The model under review builds one solid part; all positions refer to its coordinate system, in mm. Face numbers are marked on the shaded views. A direction names the side the tool comes from. Round coordinates to 2 decimals unless told otherwise and drop trailing zeros. Order: outer loops, then holes, each group sorted by start corner. A loop starts at its lowest first (then second) coordinate and runs counter-clockwise, first axis right, second up. Notation, with made-up numbers: M 78,-24.75 L 90,-24.75 A23 cw 90,14.25 Z; hole C 5,-33.75 d1. An arc over 180 degrees is marked long. Use a Markdown table: item, result. Add a question column.
1. The part is to be moulded in two halves that separate along X. For the marked faces 4, 5 and 6, say which applies: +X half, -X half, draft (parallel to the pull), parting line (faces both ways), or undercut.
2. Insertion check: P1, Ø8, axis at y = 15.5, z = 25, coming from the -X side; P2, Ø12.5, axis at x = 15.5, y = 8.5, coming from the +Z side; P3, Ø7.5, axis at y = 8, z = 25, coming from the +X side. Each pin has a flat end and moves straight along its axis. Give the tip position at first contact, or say it passes through.
3. Consider section A-A on x = 57.15. State the section outline as (y, z) points, then the cut area to 3 significant figures.
4. To check wall thickness, follow probe 1 along X at (y, z) = (12.7, 8.75); probe 2 along Y at (x, z) = (57, 9); probe 3 along Z at (x, y) = (3, 20). State the ranges of each line that lie inside material, in increasing order.
5. For the marked faces 1, 2 and 3, list the 3-axis set-ups (+Z, -Z, +X, -X, +Y, -Y) from which the entire face can be reached by the end or side of a thin tool; tool diameter is ignored.
6. Consider section B-B on y = 14.75. State the section outline as (x, z) points.
7. Consider section D-D on x = 10. State the section outline as (y, z) points.
8. Consider section C-C on z = 10. State the section outline as (x, y) points (3 decimals).
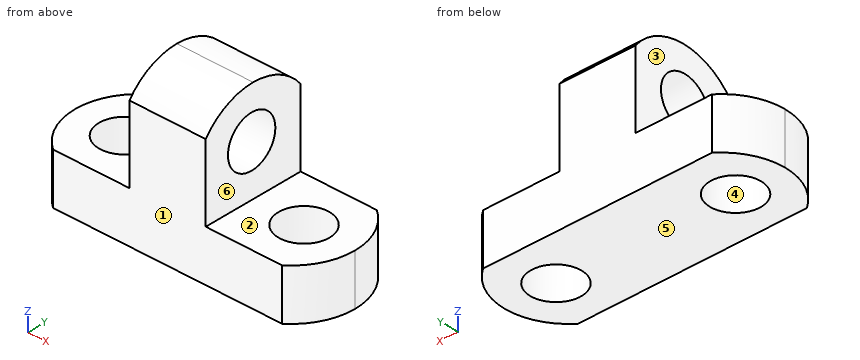
from build123d import *

# Parameters (mm, degrees)
F0_W      = 69.85
F0_H      = 38.1
F1_DEPTH  = 25.4
F2_W      = 25.4
F2_H      = 25.4
F3_DEPTH  = 25.4
F4_W      = 25.4
F4_H      = 25.4
F5_DEPTH  = 25.4
F7_DEPTH  = 25.4
F9_DEPTH  = 25.4
F11_DEPTH = 50.8
F12_R     = 6.35
F13_DEPTH = 25.4
F14_R     = 6.35
F15_DEPTH = 50.8


with BuildPart() as f1:
    # F0 (on Front) → F1 (new body)
    with BuildSketch(Plane.XZ):
        with Locations((34.925, 19.05)):
            Rectangle(F0_W, F0_H)
    extrude(amount=-F1_DEPTH)

    # F2 (on Front) → F3 (cut)
    with BuildSketch(Plane.XZ):
        with Locations((57.15, 25.4)):
            Rectangle(F2_W, F2_H)
    extrude(amount=-F3_DEPTH, mode=Mode.SUBTRACT)

    # F4 (on Front) → F5 (cut)
    with BuildSketch(Plane.XZ):
        with Locations((12.7, 25.4)):
            Rectangle(F4_W, F4_H)
    extrude(amount=-F5_DEPTH, mode=Mode.SUBTRACT)

    # F6 (on Top) → F7 (cut)
    with BuildSketch(Plane.XY):
        with BuildLine():
            ThreePointArc((63.5, 25.4), (68.174032, 19.799516), (69.85, 12.7))
            Line((69.85, 12.7), (69.85, 25.4))
            Line((69.85, 25.4), (63.5, 25.4))
        make_face()
        with BuildLine():
            ThreePointArc((69.85, 12.7), (68.174032, 5.600484), (63.5, 0))
            Line((63.5, 0), (69.85, 0))
            Line((69.85, 0), (69.85, 12.7))
        make_face()
    extrude(amount=F7_DEPTH, mode=Mode.SUBTRACT)

    # F8 (on Top) → F9 (cut)
    with BuildSketch(Plane.XY):
        with BuildLine():
            ThreePointArc((6.35, 0), (1.675968, 5.600484), (0, 12.7))
            Line((0, 12.7), (0, 0))
            Line((0, 0), (6.35, 0))
        make_face()
        with BuildLine():
            ThreePointArc((0, 12.7), (1.675968, 19.799516), (6.35, 25.4))
            Line((6.35, 25.4), (0, 25.4))
            Line((0, 25.4), (0, 12.7))
        make_face()
    extrude(amount=F9_DEPTH, mode=Mode.SUBTRACT)

    # F10 (on Right) → F11 (cut)
    with BuildSketch(Plane.YZ):
        with BuildLine():
            ThreePointArc((0, 31.75), (5.600484, 36.424032), (12.7, 38.1))
            Line((12.7, 38.1), (0, 38.1))
            Line((0, 38.1), (0, 31.75))
        make_face()
        with BuildLine():
            ThreePointArc((12.7, 38.1), (19.799516, 36.424032), (25.4, 31.75))
            Line((25.4, 31.75), (25.4, 38.1))
            Line((25.4, 38.1), (12.7, 38.1))
        make_face()
    extrude(amount=F11_DEPTH, mode=Mode.SUBTRACT)

    # F12 (on Top) → F13 (cut)
    with BuildSketch(Plane.XY):
        with Locations((12.693542, 12.295053)):
            Circle(F12_R)
        with Locations((57.15, 12.7)):
            Circle(F12_R)
    extrude(amount=F13_DEPTH, mode=Mode.SUBTRACT)

    # F14 (on Right) → F15 (cut)
    with BuildSketch(Plane.YZ):
        with Locations((12.295053, 25.406458)):
            Circle(F14_R)
    extrude(amount=F15_DEPTH, mode=Mode.SUBTRACT)


solid = f1.part
Answer block:
| question | item | result |
|---|---|---|
| 1 | face 4 | undercut |
| 1 | face 5 | draft |
| 1 | face 6 | +X half |
| 2 | P1 | x = 25.4 |
| 2 | P2 | z = 12.7 |
| 2 | P3 | x = 44.45 |
| 3 | outline | M 0,0 L 6.35,0 L 6.35,12.7 L 0,12.7 Z; M 19.05,0 L 25.4,0 L 25.4,12.7 L 19.05,12.7 Z |
| 3 | area | 161 mm^2 |
| 4 | probe 1 | 0 to 6.36, 19.03 to 50.8, 63.5 to 69.85 |
| 4 | probe 2 | 0 to 6.35, 19.05 to 25.4 |
| 4 | probe 3 | 0 to 12.7 |
| 5 | face 1 | +Z, -Z, +X, -X, -Y |
| 5 | face 2 | +Z, +X, +Y, -Y |
| 5 | face 3 | +Z, -X, +Y, -Y |
| 6 | outline | M 0.13,0 L 6.84,0 L 6.84,12.7 L 0.13,12.7 Z; M 18.55,0 L 51.14,0 L 51.14,12.7 L 44.45,12.7 L 44.45,19.55 L 25.4,19.55 L 25.4,12.7 L 18.55,12.7 Z; M 25.4,31.26 L 44.45,31.26 L 44.45,37.97 L 25.4,37.97 Z; M 63.16,0 L 69.72,0 L 69.72,12.7 L 63.16,12.7 Z |
| 7 | outline | M 0,0 L 6.54,0 L 6.54,12.7 L 0,12.7 Z; M 18.05,0 L 25.4,0 L 25.4,12.7 L 18.05,12.7 Z |
| 8 | outline | M 0,12.7 A15.875 ccw 6.35,0 L 63.5,0 A15.875 ccw 69.85,12.7 A15.875 ccw 63.5,25.4 L 6.35,25.4 A15.875 ccw Z; hole C 12.694,12.295 d12.7; hole C 57.15,12.7 d12.7 |
